Source: CAD feature listing. Evaluate the final solid. Frame: model axes, mm. Face numbers are marked on the shaded views. Round coordinates to 2 decimals unless told otherwise and drop trailing zeros. Loops run counter-clockwise (first coordinate to the right, second up) from the corner with the lowest first, then second, coordinate; pieces in that order, holes last. Notation, with made-up numbers: (66.5, 64.5) -> (78.5, 64.5) arc R13 ccw to (78.5, 81.5) -> close; hole circle Ø5 at (24, -10.75). An arc over 180 degrees is marked (long way). Put each result on its own line as item: value. Start each with the question number.
1. Material intervals for L1, parallel to Y at x = -156, z = 1.65; L2, parallel to Y at x = -154, z = 1.3; L3, parallel to Y at x = -166, z = 0.4, sorted ascending.
2. Cut plane A-A (z = 1.1). Return the cut outline in (x, y) (3 decimals).
3. Draft query along Y for the marked faces 1, 2 and 3. Return one class per face: pulls with the +Y half, pulls with the -Y half, needs draft (parallel to the pull), parting line crosses it, or undercut.
4. Contact query for flat-ended pins moving along their axis: pin 1 (4 mm diameter, centred on x = -164, y = 91.5, fed in from +Z); pin 2 (3 mm diameter, centred on x = -165.66, y = 103.94, fed in from +Z) (3 decimals); pin 3 (0.9 mm diameter, centred on x = -156, z = 1, fed in from -Y); pin 4 (1 mm diameter, centred on y = 98, z = 1, fed in from +X). Output: stop coordinate, or through.
5. Cut plane B-B (x = -165). State how many separate pieces and enclosed holes the cut face has, then the cut area to 3 significant figures.
6. Cut plane C-C (x = -169.5). Return the cut outline in (y, z).
7. Cut plane D-D (y = 113). Return the cut outline in (x, z), then the cut area to 3 significant figures.
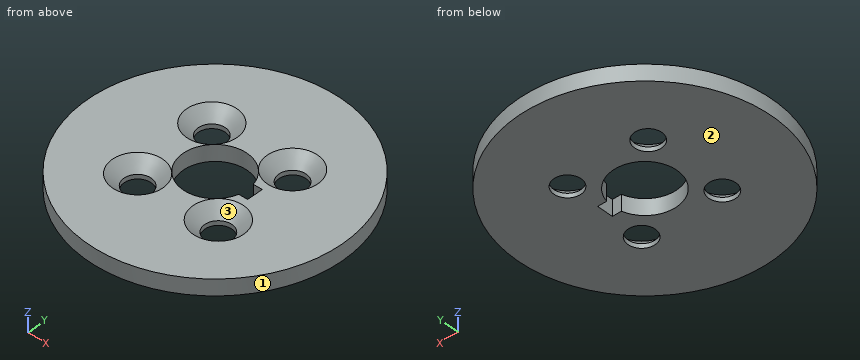
```python
from build123d import *

# Parameters (mm, degrees)
SKETCH2_R                                      = 15.875
SKETCH2_R_2                                    = 1.7
SKETCH2_R_3                                    = 4
BOSS_EXTRUDE1_DEPTH                            = 2
CSK_FOR_M3_FLAT_HEAD_MACHINE_SCREW2_AT_2_COUNT = 2
CSK_FOR_M3_FLAT_HEAD_MACHINE_SCREW2_AT_2_PITCH = 10.111626971
CSK_FOR_M3_FLAT_HEAD_MACHINE_SCREW2_AT_3_COUNT = 2
CSK_FOR_M3_FLAT_HEAD_MACHINE_SCREW2_AT_3_PITCH = 14.3
CSK_FOR_M3_FLAT_HEAD_MACHINE_SCREW2_AT_4_COUNT = 2
CSK_FOR_M3_FLAT_HEAD_MACHINE_SCREW2_AT_4_PITCH = 10.111626971
SKETCH5_W                                      = 1.314472485
SKETCH5_H                                      = 2
CUT_EXTRUDE1_DEPTH                             = 3


with BuildPart() as part:
    # Sketch2 → Boss-Extrude1 (new body)
    with BuildSketch(Plane.XY):
        with Locations((-160.606756626, 98.885631483)):
            Circle(SKETCH2_R)
        with Locations((-165.662570112, 103.941444968)):
            Circle(SKETCH2_R_2, mode=Mode.SUBTRACT)
        with Locations((-155.550943141, 103.941444968)):
            Circle(SKETCH2_R_2, mode=Mode.SUBTRACT)
        with Locations((-155.550943141, 93.829817997)):
            Circle(SKETCH2_R_2, mode=Mode.SUBTRACT)
        with Locations((-165.662570112, 93.829817997)):
            Circle(SKETCH2_R_2, mode=Mode.SUBTRACT)
        with Locations((-160.606756626, 98.885631483)):
            Circle(SKETCH2_R_3, mode=Mode.SUBTRACT)
    extrude(amount=BOSS_EXTRUDE1_DEPTH)

    # Sketch4 → CSK for M3 Flat Head Machine Screw2 (revolve, cut)
    with BuildSketch(Plane(origin=(-165.662570112, 103.941444968, 2), x_dir=(0, -1, 0), z_dir=(1, 0, 0))):
        Polygon((0, 0), (0, 2), (1.7, 2), (1.7, 1.45), (3.15, 0), align=None)
    csk_for_m3_flat_head_machine_screw2 = revolve(axis=Axis((-165.662570112, 103.941444968, 8.35), (0, 0, -1)), mode=Mode.SUBTRACT)

    # CSK for M3 Flat Head Machine Screw2 at 2: CSK for M3 Flat Head Machine Screw2 ×2
    with Locations(*[(i * CSK_FOR_M3_FLAT_HEAD_MACHINE_SCREW2_AT_2_PITCH, 0, 0) for i in range(1, CSK_FOR_M3_FLAT_HEAD_MACHINE_SCREW2_AT_2_COUNT)]):
        add(csk_for_m3_flat_head_machine_screw2, mode=Mode.SUBTRACT)

    # CSK for M3 Flat Head Machine Screw2 at 3: CSK for M3 Flat Head Machine Screw2 ×2
    with Locations(*[Vector(0.707106781, -0.707106781, 0) * (i * CSK_FOR_M3_FLAT_HEAD_MACHINE_SCREW2_AT_3_PITCH) for i in range(1, CSK_FOR_M3_FLAT_HEAD_MACHINE_SCREW2_AT_3_COUNT)]):
        add(csk_for_m3_flat_head_machine_screw2, mode=Mode.SUBTRACT)

    # CSK for M3 Flat Head Machine Screw2 at 4: CSK for M3 Flat Head Machine Screw2 ×2
    with Locations(*[(0, -i * CSK_FOR_M3_FLAT_HEAD_MACHINE_SCREW2_AT_4_PITCH, 0) for i in range(1, CSK_FOR_M3_FLAT_HEAD_MACHINE_SCREW2_AT_4_COUNT)]):
        add(csk_for_m3_flat_head_machine_screw2, mode=Mode.SUBTRACT)

    # Sketch5 → Cut-Extrude1 (cut, through all)
    with BuildSketch(Plane(origin=(0, 0, 0), x_dir=(-1, 0, 0), z_dir=(0, 0, -1))):
        with Locations((156.263992868, 98.885631483)):
            Rectangle(SKETCH5_W, SKETCH5_H)
    extrude(amount=-CUT_EXTRUDE1_DEPTH, mode=Mode.SUBTRACT)


solid = part.part
```
Solution:
1. L1: y = 83.69 to 91.07, 96.59 to 97.89, 99.89 to 101.18, 106.71 to 114.08
1. L2: y = 84.45 to 91.93, 95.73 to 102.04, 105.84 to 113.32
1. L3: y = 83.95 to 92.16, 95.5 to 102.28, 105.61 to 113.82
2. outline: circle Ø31.75 at (-160.607, 98.886); hole circle Ø4.5 at (-165.663, 93.83); hole circle Ø4.5 at (-165.663, 103.941); hole circle Ø4.5 at (-155.551, 93.83); hole circle Ø4.5 at (-155.551, 103.941); hole (-156.734, 97.886) -> (-155.607, 97.886) -> (-155.607, 99.886) -> (-156.734, 99.886) arc R4 ccw (long way) to start
3. face 1: parting line crosses it
3. face 2: needs draft
3. face 3: undercut
4. pin 1: stops at z = 2
4. pin 2: passes through
4. pin 3: stops at y = 83.56
4. pin 4: stops at x = -144.74
5. separate pieces: 3
5. enclosed holes: 0
5. area: 44.1 mm^2
6. outline: (85.74, 0) -> (112.04, 0) -> (112.04, 2) -> (85.74, 2) -> close
7. outline: (-167.87, 0) -> (-153.34, 0) -> (-153.34, 2) -> (-167.87, 2) -> close
7. area: 29.1 mm^2
